```python
from build123d import *

# Parameters (mm, degrees)
SKETCH1_R           = 4
BOSS_EXTRUDE1_DEPTH = 20
SKETCH2_R           = 1
SKETCH2_R_2         = 0.5
BOSS_EXTRUDE2_DEPTH = 0.5
SKETCH4_R           = 0.5
BOSS_EXTRUDE3_DEPTH = 5
FILLET2_R           = 0.1
SKETCH5_R           = 0.25
CUT_EXTRUDE1_DEPTH  = 21.784609691


with BuildPart() as part:
    # Sketch1 → Boss-Extrude1 (new body)
    with BuildSketch(Plane.XY):
        Circle(SKETCH1_R)
    extrude(amount=BOSS_EXTRUDE1_DEPTH)

    # Sketch2 → Boss-Extrude2 (add)
    with BuildSketch(Plane.XY.offset(20)):
        Circle(SKETCH2_R)
        Circle(SKETCH2_R_2, mode=Mode.SUBTRACT)
    extrude(amount=BOSS_EXTRUDE2_DEPTH)

    # Sketch4 → Boss-Extrude3 (add)
    with BuildSketch(Plane.XY.offset(20)):
        Circle(SKETCH4_R)
    extrude(amount=BOSS_EXTRUDE3_DEPTH)

    # Fillet2
    fillet2_edges = [part.edges().sort_by_distance(p)[0] for p in [
        (-1, 0, 20.5),
    ]]
    fillet(fillet2_edges, radius=FILLET2_R)

    # Sketch5 → Cut-Extrude1 (cut, through all)
    with BuildSketch(Plane.XY.offset(20)):
        with Locations((0, 3)):
            Circle(SKETCH5_R)
        with Locations(Location((0, -3, 0), (0, 0, 180))):
            Circle(SKETCH5_R)
        with Locations((3, 0)):
            Circle(SKETCH5_R)
        with Locations(Location((-3, 0, 0), (0, 0, 180))):
            Circle(SKETCH5_R)
    extrude(amount=-CUT_EXTRUDE1_DEPTH, mode=Mode.SUBTRACT)


solid = part.part
```
Check sheet for the modelled part. Datum: model origin and axes. Units: mm. A direction names the side the tool comes from. Round coordinates to 2 decimals unless told otherwise and drop trailing zeros. Order: outer loops, then holes, each group sorted by start corner. A loop starts at its lowest first (then second) coordinate and runs counter-clockwise, first axis right, second up.
1) Scan lines: line 1 (Y direction, x = 0, z = 15.25); line 2 (Z direction, x = -1.25, y = 0); line 3 (Y direction, x = -3, z = 5.75). Record each from-to range of solid material in increasing order.
2) Section check A-A (x = 3). Record the boundary of the cut face in (y, z).
3) Section check B-B (z = 1.5). Record the boundary of the cut face in (x, y), and give its area (3 significant figures).
4) Go/stop test with flat-tipped pins: pin 1 Ø2 at (x, z) = (0.5, 5) entering from +Y; pin 2 Ø3 at (x, y) = (1.5, 2.5) entering from +Z; pin 3 Ø1.5 at (y, z) = (-2, 9) entering from +X. Record where each tip stops, or that it passes through.
5) Section check C-C (y = 0). Record the boundary of the cut face in (x, z).
6) Tool access check on faces 1 (the flat face through (1, -1, 20)), 2 (the flat face through (0, 0, 25)). Record the directions out of +Z, -Z, +X, -X, +Y, -Y that give a thin tool (end or side, any length) a straight path to the whole face; none if there is none.
Result:
1. line 1: y = -4 to -3.25, -2.75 to 2.75, 3.25 to 4
1. line 2: z = 0 to 20
1. line 3: y = -2.65 to -0.25, 0.25 to 2.65
2. outline: (-2.65, 0) - (-0.25, 0) - (-0.25, 20) - (-2.65, 20) - close; (0.25, 0) - (2.65, 0) - (2.65, 20) - (0.25, 20) - close
3. outline: circle Ø8 at (0, 0); hole circle Ø0.5 at (-3, 0); hole circle Ø0.5 at (0, -3); hole circle Ø0.5 at (0, 3); hole circle Ø0.5 at (3, 0)
3. area: 49.5 mm2
4. pin 1: stops at y = 4
4. pin 2: stops at z = 20
4. pin 3: stops at x = 3.8
5. outline: (-4, 0) - (-3.25, 0) - (-3.25, 20) - (-4, 20) - close; (-2.75, 0) - (2.75, 0) - (2.75, 20) - (1, 20) - (1, 20.4) arc R0.1 ccw to (0.9, 20.5) - (0.5, 20.5) - (0.5, 25) - (-0.5, 25) - (-0.5, 20.5) - (-0.9, 20.5) arc R0.1 ccw to (-1, 20.4) - (-1, 20) - (-2.75, 20) - close; (3.25, 0) - (4, 0) - (4, 20) - (3.25, 20) - close
6. face 1: +Z
6. face 2: +Z, +X, -X, +Y, -Y
